Geometry check sheet. Reference: drawing and pictorial views, mm from the part's lowest x, y, z. A direction names the side the tool comes from. Coordinates: 2 decimals unless noted, no trailing zeros. Loops run counter-clockwise (first coordinate to the right, second up) from the corner with the lowest first, then second, coordinate; pieces in that order, holes last. Notation, with made-up numbers: (80.5, -28.75) -> (101.5, -28.75) arc R20 cw to (101.5, -6.75) -> close; hole circle Ø7 at (79, 47). An arc over 180 degrees is marked (long way). Answer as a JSON object with one key per item and string values.
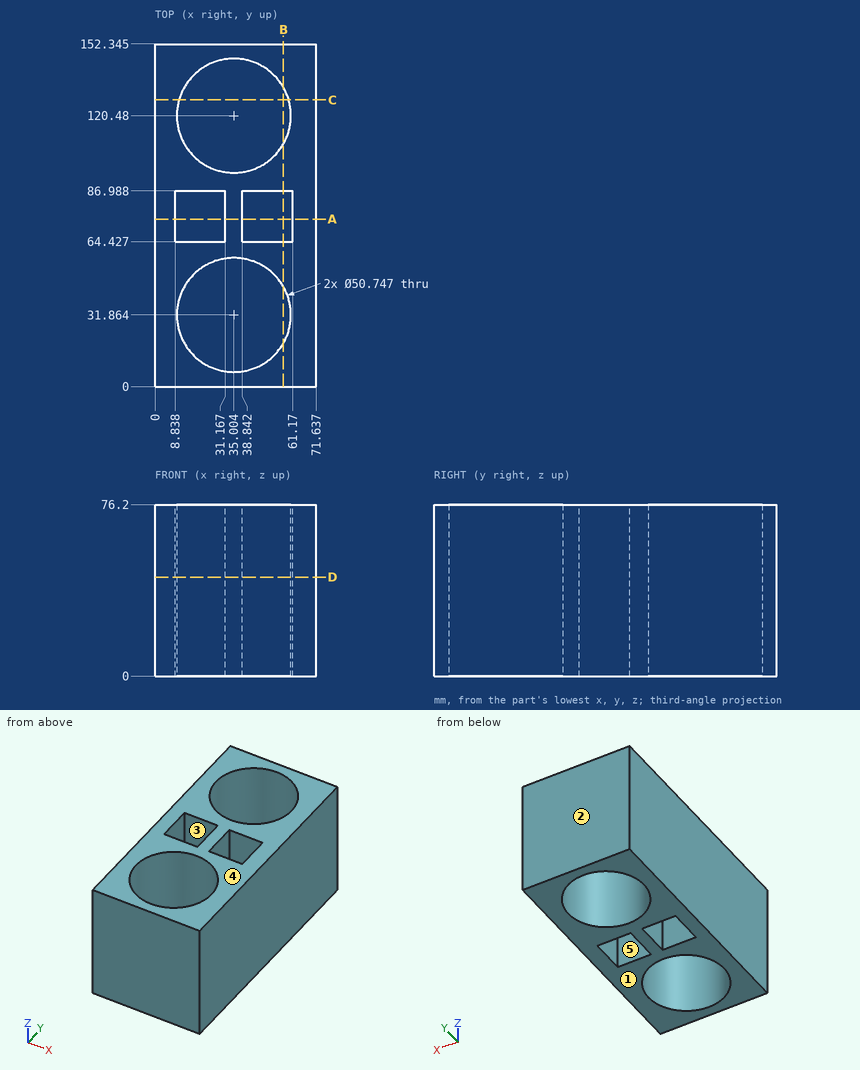
1. Thickness scan on probe 1 along X at (y, z) = (82.5, 26); probe 2 along Y at (x, z) = (25.5, 68.5) (1 decimal); probe 3 along Y at (x, z) = (55, 57) (1 decimal). Record the ranges inside material, lowest first. Write a range as from..to.
Evaluation:
{"probe 1": "x = 0..8.84, 31.17..38.84, 61.17..71.64", "probe 2": "y = 0..8.3, 55.4..64.4, 87..97, 144..152.3", "probe 3": "y = 0..16.2, 47.5..64.4, 87..104.9, 136.1..152.3"}
2. Section check D-D, the plane z = 44. Record the boundary of the cut face in (x, y) (1 decimal).
Evaluation:
{"outline": "(0, 0) -> (71.6, 0) -> (71.6, 152.3) -> (0, 152.3) -> close; hole (8.8, 64.4) -> (31.2, 64.4) -> (31.2, 87) -> (8.8, 87) -> close; hole circle Ø50.7 at (35, 31.9); hole circle Ø50.7 at (35, 120.5); hole (38.8, 64.4) -> (61.2, 64.4) -> (61.2, 87) -> (38.8, 87) -> close"}
3. Section check C-C, the plane y = 127.5. Record the boundary of the cut face in (x, z), then the cut area to 3 significant figures.
Evaluation:
{"outline": "(0, 0) -> (10.62, 0) -> (10.62, 76.2) -> (0, 76.2) -> close; (59.39, 0) -> (71.64, 0) -> (71.64, 76.2) -> (59.39, 76.2) -> close", "area": "1,740 mm^2"}
4. Section check A-A, the plane y = 74.5. Record the boundary of the cut face in (x, z).
Evaluation:
{"outline": "(0, 0) -> (8.84, 0) -> (8.84, 76.2) -> (0, 76.2) -> close; (31.17, 0) -> (38.84, 0) -> (38.84, 76.2) -> (31.17, 76.2) -> close; (61.17, 0) -> (71.64, 0) -> (71.64, 76.2) -> (61.17, 76.2) -> close"}
5. Tool access check on the marked faces 4 and 5. Record the directions out of +Z, -Z, +X, -X, +Y, -Y that give a thin tool (end or side, any length) a straight path to the whole face; none if there is none.
Evaluation:
{"face 4": "+Z, +X, -X, +Y, -Y", "face 5": "+Z, -Z"}
6. Depth check by flat-ended pin: P1, Ø24.5, axis at x = 24.5, z = 38, coming from the -Y side. Enter the tip coordinate at first touch or a pass-through.
Evaluation:
{"P1": "stops at y = 0"}
7. Mould release check, pull along Y, two halves, no side actions. Record for the marked faces 1, 2 and 3: released by +Y, released by -Y, zero draft, split by the parting line, or undercut.
Evaluation:
{"face 1": "zero draft", "face 2": "released by +Y", "face 3": "undercut"}
8. Section check B-B, the plane x = 57. Record the boundary of the cut face in (y, z) (1 decimal).
Evaluation:
{"outline": "(0, 0) -> (19.2, 0) -> (19.2, 76.2) -> (0, 76.2) -> close; (44.5, 0) -> (64.4, 0) -> (64.4, 76.2) -> (44.5, 76.2) -> close; (87, 0) -> (107.8, 0) -> (107.8, 76.2) -> (87, 76.2) -> close; (133.1, 0) -> (152.3, 0) -> (152.3, 76.2) -> (133.1, 76.2) -> close"}
